```python
from build123d import *

# Parameters (mm, degrees)
F0_W     = 59.4862774014
F0_H     = 38.7252047658
F1_DEPTH = 44.196
F2_R     = 7.9122216874
F3_DEPTH = 70.104
F4_R     = 5.08
F5_SIZE  = 5.07999


# Not quite as in the source:
# - a fillet or chamfer is up to 0.001 mm smaller than in the source, because OpenCascade refuses the exact size


with BuildPart() as f1:
    # F0 (on Front) → F1 (new body)
    with BuildSketch(Plane.XZ):
        with Locations((29.7431387007, 19.3626023829)):
            Rectangle(F0_W, F0_H)
    extrude(amount=F1_DEPTH)

    # F2 (on face) → F3 (cut)
    with BuildSketch(Plane.XZ.offset(44.196)):
        with Locations((17.7647974342, 13.3899012581)):
            Circle(F2_R)
    extrude(amount=-F3_DEPTH, mode=Mode.SUBTRACT)

    # F4
    f4_edges = [f1.edges().sort_by_distance(p)[0] for p in [
        (59.486277, -22.098, 38.725205),
        (59.486277, -22.098, 0),
        (59.486277, 0, 19.362602),
        (29.743139, 0, 38.725205),
        (29.743139, 0, 0),
    ]]
    fillet(f4_edges, radius=F4_R)

    # F5 (size 5.08 in the source; OpenCascade refuses exactly that, so slightly less here)
    f5_edges = [f1.edges().sort_by_distance(p)[0] for p in [
        (0, -44.196, 19.362602),
        (27.203139, -44.196, 0),
        (0, -24.638, 0),
    ]]
    chamfer(f5_edges, length=F5_SIZE)


solid = f1.part
```
Part model, mm, in its own coordinate system. Coordinates: 2 decimals unless noted, no trailing zeros. Order: outer loops, then holes, each group sorted by start corner. A loop starts at its lowest first (then second) coordinate and runs counter-clockwise, first axis right, second up. Notation, with made-up numbers: (57.5, 60) - (109.5, 60) arc R24 cw to (109.5, 71) - close; hole circle Ø9 at (-30.5, -21). An arc over 180 degrees is marked (long way). Return JSON: item names as keys, results as strings. Group by question number.
Item 1: Cut at A-A (x = 20.5). List the corners of the cut face in (y, z).
Item 2: Cut at D-D (x = 46). List the corners of the cut face in (y, z), plus the area to 3 significant figures.
Item 3: Cut at B-B (z = 8). List the corners of the cut face in (x, y).
Item 4: Cut at C-C (y = -42). List the corners of the cut face in (x, z), plus the area to 3 significant figures.
Item 5: Pull direction Z, two halves, no side cores. Call faces 1 (the face through (57.96, -22.34, 1.45)), 2 (the face through (30.09, -1.53, 37.28)), 3 (the face through (29, -44.196, 20)), 4 (the face through (9.86, -22.41, 13.74)): pulls with the +Z half, pulls with the -Z half, needs draft (parallel to the pull), parting line crosses it, or undercut.
Item 6: Drill centre lines: probe 1 along X at (y, z) = (-25, 17); probe 2 along Z at (x, y) = (21.5, -28.5); probe 3 along Z at (x, y) = (24, -33.5). Where is each one in solid material? Low to high. Write a range as from..to.
Check values:
{
 "1": {"outline": "(-44.2, 5.08) - (-39.12, 0) - (-5.08, 0) arc R5.08 ccw to (0, 5.08) - (0, 5.97) - (-44.2, 5.97) - close; (-44.2, 20.81) - (0, 20.81) - (0, 33.65) arc R5.08 ccw to (-5.08, 38.73) - (-39.12, 38.73) - (-44.2, 33.65) - close"},
 "2": {"outline": "(-44.2, 5.08) - (-39.12, 0) - (-5.08, 0) arc R5.08 ccw to (0, 5.08) - (0, 33.65) arc R5.08 ccw to (-5.08, 38.73) - (-39.12, 38.73) - (-44.2, 33.65) - close", "area": "1,670 mm2"},
 "3": {"outline": "(0, -39.12) - (5.08, -44.2) - (11.97, -44.2) - (11.97, 0) - (5.08, 0) - (0, -5.08) - close; (23.56, -44.2) - (54.41, -44.2) - (59.49, -39.12) - (59.49, -5.08) arc R5.08 ccw to (54.41, 0) - (23.56, 0) - close"},
 "4": {"outline": "(2.88, 5.08) - (5.08, 2.88) - (54.41, 2.88) arc R2.2 ccw to (56.6, 5.08) - (56.6, 33.65) arc R2.2 ccw to (54.41, 35.84) - (5.08, 35.84) - (2.88, 33.65) - close; hole circle Ø15.82 at (17.76, 13.39)", "area": "1,570 mm2"},
 "5": {"face 1": "pulls with the -Z half", "face 2": "pulls with the +Z half", "face 3": "needs draft", "face 4": "undercut"},
 "6": {"probe 1": "x = 0..10.72, 24.81..59.49", "probe 2": "z = 0..6.41, 20.36..38.73", "probe 3": "z = 0..8.52, 18.26..38.73"}
}
